from build123d import *

# Parameters (mm, degrees)
SKETCH1_W           = 79.2
SKETCH1_H           = 79.2
BOSS_EXTRUDE1_DEPTH = 3
CUT_EXTRUDE1_DEPTH  = 3
SKETCH3_W           = 3
SKETCH3_H           = 79.2
BOSS_EXTRUDE2_DEPTH = 88.9
CUT_EXTRUDE2_DEPTH  = 88.9
SKETCH5_R           = 7.5
CUT_EXTRUDE3_DEPTH  = 88.9
SKETCH6_W           = 12
SKETCH6_H           = 15
CUT_EXTRUDE4_DEPTH  = 88.9
FILLET1_R           = 2.5


with BuildPart() as part:
    # Sketch1 → Boss-Extrude1 (new body)
    with BuildSketch(Plane(origin=(0, 0, 0), x_dir=(1, 0, 0), z_dir=(0, 1, 0))):
        Rectangle(SKETCH1_W, SKETCH1_H)
    extrude(amount=BOSS_EXTRUDE1_DEPTH)

    # Sketch2 → Cut-Extrude1 (cut)
    with BuildSketch(Plane(origin=(0, 3, 0), x_dir=(1, 0, 0), z_dir=(0, 1, 0))):
        with BuildLine():
            Line((-20.4, -25.4), (20.4, -25.4))
            ThreePointArc((20.4, -25.4), (23.935533906, -23.935533906), (25.4, -20.4))
            Line((25.4, -20.4), (25.4, 20.4))
            ThreePointArc((25.4, 20.4), (23.935533906, 23.935533906), (20.4, 25.4))
            Line((20.4, 25.4), (-20.4, 25.4))
            ThreePointArc((-20.4, 25.4), (-23.935533906, 23.935533906), (-25.4, 20.4))
            Line((-25.4, 20.4), (-25.4, -20.4))
            ThreePointArc((-25.4, -20.4), (-23.935533906, -23.935533906), (-20.4, -25.4))
        make_face()
    extrude(amount=-CUT_EXTRUDE1_DEPTH, mode=Mode.SUBTRACT)

    # Sketch3 → Boss-Extrude2 (add)
    with BuildSketch(Plane(origin=(0, 3, 0), x_dir=(1, 0, 0), z_dir=(0, 1, 0))):
        with Locations((-38.1, 0)):
            Rectangle(SKETCH3_W, SKETCH3_H)
        with Locations((38.1, 0)):
            Rectangle(SKETCH3_W, SKETCH3_H)
    extrude(amount=BOSS_EXTRUDE2_DEPTH)

    # Sketch4 → Cut-Extrude2 (cut)
    with BuildSketch(Plane(origin=(39.6, 0, 0), x_dir=(0, 0, -1), z_dir=(1, 0, 0))):
        Polygon((-39.6, 0), (-9.739879916, 91.9), (-41.709880552, 102.287682895), (-62.726275387, 13.336826297), align=None)
        Polygon((39.6, 0), (9.739879916, 91.9), (57.349998408, 101.564802913), align=None)
    extrude(amount=-CUT_EXTRUDE2_DEPTH, mode=Mode.SUBTRACT)

    # Sketch5 → Cut-Extrude3 (cut)
    with BuildSketch(Plane(origin=(39.6, 0, 0), x_dir=(0, 0, -1), z_dir=(1, 0, 0))):
        with Locations((0, 79.9)):
            Circle(SKETCH5_R)
    extrude(amount=-CUT_EXTRUDE3_DEPTH, mode=Mode.SUBTRACT)

    # Sketch6 → Cut-Extrude4 (cut)
    with BuildSketch(Plane.ZY.offset(39.6)):
        with Locations((0, 87.4)):
            Rectangle(SKETCH6_W, SKETCH6_H)
    extrude(amount=-CUT_EXTRUDE4_DEPTH, mode=Mode.SUBTRACT)

    # Fillet1
    # the kernel refuses this fillet: 2.5 mm, written as the material it takes off along each edge
    with BuildSketch(Plane(origin=(45.85, 91.9, 6), x_dir=(0, 0, 1), z_dir=(-1, 0, 0)), Plane(origin=(-30.35, 91.9, -6), x_dir=(0, -1, 0), z_dir=(-1, 0, 0))) as fillet1_piece_1:
        with BuildLine():
            CenterArc((FILLET1_R, -FILLET1_R), FILLET1_R, 90, 90)
            Line((0, -FILLET1_R), (0, 0))
            Line((0, 0), (FILLET1_R, 0))
        make_face()
    extrude(amount=15.5, mode=Mode.SUBTRACT)
    with BuildSketch(Plane(origin=(44.1408908, 91.9, 9.739879916), x_dir=(0, 0, -1), z_dir=(-1, 0, 0)), Plane(origin=(-32.0591092, 91.9, 9.739879916), x_dir=(0, 0, -1), z_dir=(-1, 0, 0))) as fillet1_piece_2:
        with BuildLine():
            CenterArc((FILLET1_R * 0.726542528005, FILLET1_R), FILLET1_R, 198, 72)
            Line((-FILLET1_R * 0.22451398829, FILLET1_R * 0.690983005625), (0, 0))
            Line((0, 0), (FILLET1_R * 0.726542528005, 0))
        make_face()
    extrude(amount=12.0817816, mode=Mode.SUBTRACT)
    with BuildSketch(Plane(origin=(30.35, 91.9, -6), x_dir=(0, -1, 0), z_dir=(1, 0, 0)), Plane(origin=(-45.85, 91.9, 6), x_dir=(0, 0, 1), z_dir=(1, 0, 0))) as fillet1_piece_3:
        with BuildLine():
            CenterArc((FILLET1_R, FILLET1_R), FILLET1_R, 180, 90)
            Line((0, FILLET1_R), (0, 0))
            Line((0, 0), (FILLET1_R, 0))
        make_face()
    extrude(amount=15.5, mode=Mode.SUBTRACT)
    with BuildSketch(Plane(origin=(44.1408908, 91.9, -9.739879916), x_dir=(0, 0, 1), z_dir=(-1, 0, 0)), Plane(origin=(-32.0591092, 91.9, -9.739879916), x_dir=(0, 0, 1), z_dir=(-1, 0, 0))) as fillet1_piece_4:
        with BuildLine():
            CenterArc((FILLET1_R * 0.726542528005, -FILLET1_R), FILLET1_R, 90, 72)
            Line((-FILLET1_R * 0.22451398829, -FILLET1_R * 0.690983005625), (0, 0))
            Line((0, 0), (FILLET1_R * 0.726542528005, 0))
        make_face()
    extrude(amount=12.0817816, mode=Mode.SUBTRACT)


solid = part.part
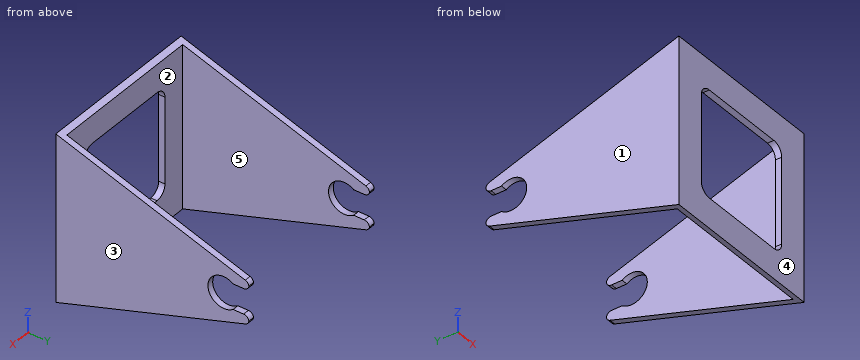
Model file for the job. Use its own axes, mm. Face numbers are marked on the shaded views. A direction names the side the tool comes from. Give positions to 0.01 mm unless a question says otherwise; leave off trailing zeros. Order: outer loops, then holes, each group sorted by start corner. A loop starts at its lowest first (then second) coordinate and runs counter-clockwise, first axis right, second up. Notation, with made-up numbers: (59, 49) - (96, 49) arc R8 cw to (96, 57) - close; hole circle Ø4 at (67.25, 64). An arc over 180 degrees is marked (long way). Write item = value, one per line. Start each with the question number.
1. Drop flat-ended pins along their axis: P1, Ø0.9, axis at x = 10, y = 1, coming from the -Z side; P2, Ø1.5, axis at x = -3.5, y = 1.5, coming from the +Z side; P3, Ø2.5, axis at x = -38.5, y = 87, coming from the +Z side; P4, Ø13.5, axis at y = 79.9, z = 0, coming from the +X side. Give the stop position or say it passes through.
2. Cut at C-C, the plane z = 0. List the corners of the cut face in (x, y), and give its area (3 significant figures).
3. Cut at A-A, the plane x = -1. List the corners of the cut face in (y, z).
4. Which spindle directions (+Z, -Z, +X, -X, +Y, -Y) get a long thin tool onto all of the face, cutting with end or side? Do the marked faces 4 and 5. Say none if no direction does.
5. Cut at B-B, the plane y = 18. List the corners of the cut face in (x, z), and give its area (3 significant figures).
6. Two-plate mould, pull along X, no slides. Class the marked faces 1, 2 and 3: pulls with the +X half, pulls with the -X half, needs draft (parallel to the pull), parting line crosses it, or undercut.
7. Probe line 1 along X through (y, z) = (51, -17); line 2 along Y through (x, z) = (37, 0); line 3 along Z through (x, y) = (-37.95, 79.9). List the from-to ranges inside material, lowest first.
8. Cut at D-D, the plane y = 79.9. List the corners of the cut face in (x, z), and give its area (3 significant figures).
Taken from the geometry:
q1.P1 = -39.42
q1.P2 = 39.36
q1.P3 = 11.74
q1.P4 = through
q2.outline = (-39.6, 0) - (-25.4, 0) - (-25.4, 3) - (-36.6, 3) - (-36.6, 72.4) - (-39.6, 72.4) - close; (25.4, 0) - (39.6, 0) - (39.6, 72.4) - (36.6, 72.4) - (36.6, 3) - (25.4, 3) - close
q2.area = 502 mm²
q3.outline = (0, -39.6) - (3, -38.63) - (3, -25.4) - (0, -25.4) - close; (0, 25.4) - (3, 25.4) - (3, 38.63) - (0, 39.6) - close
q4.face_4 = +Z, -Z, +X, -X, -Y
q4.face_5 = +Z, -Z, +Y
q5.outline = (-39.6, -33.75) - (-36.6, -33.75) - (-36.6, 33.75) - (-39.6, 33.75) - close; (36.6, -33.75) - (39.6, -33.75) - (39.6, 33.75) - (36.6, 33.75) - close
q5.area = 405 mm²
q6.face_1 = pulls with the -X half
q6.face_2 = undercut
q6.face_3 = pulls with the +X half
q7.line_1 = -39.6 to -36.6, 36.6 to 39.6
q7.line_2 = 0 to 72.4
q7.line_3 = -13.64 to -7.5, 7.5 to 13.64
q8.outline = (-39.6, -13.64) - (-36.6, -13.64) - (-36.6, -7.5) - (-39.6, -7.5) - close; (-39.6, 7.5) - (-36.6, 7.5) - (-36.6, 13.64) - (-39.6, 13.64) - close; (36.6, -13.64) - (39.6, -13.64) - (39.6, -7.5) - (36.6, -7.5) - close; (36.6, 7.5) - (39.6, 7.5) - (39.6, 13.64) - (36.6, 13.64) - close
q8.area = 73.7 mm²
